from build123d import *

# Parameters (mm, degrees)
SKETCH1_R               = 10
BOSS_EXTRUDE1_DEPTH     = 35
SKETCH2_R               = 15
BOSS_EXTRUDE2_DEPTH     = 10
SKETCH3_R               = 2.5
BOSS_EXTRUDE3_DEPTH     = 5
CUT_EXTRUDE1_DEPTH      = 50
CUT_EXTRUDE1_DEPTH_BACK = 26
SKETCH7_R               = 2.5


with BuildPart() as part:
    # Sketch1 → Boss-Extrude1 (new body)
    with BuildSketch(Plane(origin=(0, 0, 0), x_dir=(1, 0, 0), z_dir=(0, 1, 0))):
        with Locations(Location((0, 0, 0), (0, 0, 270))):
            Circle(SKETCH1_R)
    extrude(amount=BOSS_EXTRUDE1_DEPTH)

    # Sketch2 → Boss-Extrude2 (add)
    with BuildSketch(Plane(origin=(0, 35, 0), x_dir=(1, 0, 0), z_dir=(0, 1, 0))):
        with Locations(Location((0, 0, 0), (0, 0, 270))):
            Circle(SKETCH2_R)
    extrude(amount=BOSS_EXTRUDE2_DEPTH)

    # Sketch3 → Boss-Extrude3 (add)
    with BuildSketch(Plane(origin=(0, 45, 0), x_dir=(1, 0, 0), z_dir=(0, 1, 0))):
        with BuildLine():
            Line((-60, 0), (-60, 12.589573297))
            Line((-60, 12.589573297), (-17.498503567, 12.589573297))
            ThreePointArc((-17.498503567, 12.589573297), (-13.964027799, 14.053601095), (-12.5, 17.588076863))
            Line((-12.5, 17.588076863), (-12.5, 60))
            Line((-12.5, 60), (12.589573297, 60))
            Line((12.589573297, 60), (12.589573297, 17.498503567))
            ThreePointArc((12.589573297, 17.498503567), (14.053601095, 13.964027799), (17.588076863, 12.5))
            Line((17.588076863, 12.5), (60, 12.5))
            Line((60, 12.5), (60, -12.589573297))
            Line((60, -12.589573297), (17.498503567, -12.589573297))
            ThreePointArc((17.498503567, -12.589573297), (13.964027799, -14.053601095), (12.5, -17.588076863))
            Line((12.5, -17.588076863), (12.5, -60))
            Line((12.5, -60), (-12.589573297, -60))
            Line((-12.589573297, -60), (-12.589573297, -17.498503567))
            ThreePointArc((-12.589573297, -17.498503567), (-14.053601095, -13.964027799), (-17.588076863, -12.5))
            Line((-17.588076863, -12.5), (-60, -12.5))
            Line((-60, -12.5), (-60, 0))
        make_face()
        with Locations(Location((0, 40, 0), (0, 0, 270))):
            Circle(SKETCH3_R, mode=Mode.SUBTRACT)
        with Locations(Location((40, 0, 0), (0, 0, 270))):
            Circle(SKETCH3_R, mode=Mode.SUBTRACT)
        with Locations(Location((0, -40, 0), (0, 0, 270))):
            Circle(SKETCH3_R, mode=Mode.SUBTRACT)
        with Locations(Location((-40, 0, 0), (0, 0, 270))):
            Circle(SKETCH3_R, mode=Mode.SUBTRACT)
    extrude(amount=BOSS_EXTRUDE3_DEPTH)

    # Sketch7 → Cut-Extrude1 (cut, two sides: drawn at the far end of the back side and taken through both)
    with BuildSketch(Plane.XY.offset(-CUT_EXTRUDE1_DEPTH_BACK)):
        with Locations(Location((0, 16.5, 0), (0, 0, 90.000000004))):
            Circle(SKETCH7_R)
    extrude(amount=CUT_EXTRUDE1_DEPTH + CUT_EXTRUDE1_DEPTH_BACK, mode=Mode.SUBTRACT)


solid = part.part
Could you check a few things on this model? Use its own coordinates, in mm. A direction names the side the tool comes from. Round coordinates to 2 decimals unless told otherwise and drop trailing zeros. Loops run counter-clockwise (first coordinate to the right, second up) from the corner with the lowest first, then second, coordinate; pieces in that order, holes last. Notation, with made-up numbers: (63.5, -23.75) - (106.5, -23.75) arc R26 cw to (106.5, 11.25) - close; hole circle Ø4 at (2.25, 64). An arc over 180 degrees is marked (long way). Write item = value, one per line.
1) Imagine slicing it at B-B (z = 0). Please give me the cut outline in (x, y), and give its area (3 significant figures).
Computed:
outline = (-60, 45) - (-42.5, 45) - (-42.5, 50) - (-60, 50) - close; (-37.5, 45) - (-15, 45) - (-15, 35) - (-10, 35) - (-10, 0) - (10, 0) - (10, 35) - (15, 35) - (15, 45) - (37.5, 45) - (37.5, 50) - (-37.5, 50) - close; (42.5, 45) - (60, 45) - (60, 50) - (42.5, 50) - close; hole circle Ø5 at (0, 16.5)
area = 1,530 mm2
2) On a 3-axis mill with a long thin cutter (end or side, diameter ignored), from which of +Z, -Z, +X, -X, +Y, -Y can I reach the whole of each face in a straight line? I mean faces 1 (the flat face through (39, 47, 12.59)), 2 (the flat face through (-38, 47, 12.5)), 3 (the flat face through (12.59, 47, -39)), 4 (the flat face through (-12.5, 47, -38)). Say none if no direction works.
Computed:
face_1 = +Z, +X, +Y, -Y
face_2 = +Z, -X, +Y, -Y
face_3 = -Z, +X, +Y, -Y
face_4 = -Z, -X, +Y, -Y
3) Imagine slicing it at A-A (x = -40). Please give me the cut outline in (y, z).
Computed:
outline = (45, -12.59) - (50, -12.59) - (50, -2.5) - (45, -2.5) - close; (45, 2.5) - (50, 2.5) - (50, 12.5) - (45, 12.5) - close
4) I need wall thicknesses on line 1 along X through (y, z) = (46.65, 0); line 2 along X through (y, z) = (47, 50.5); line 3 along Y through (x, z) = (0, 1). Which ranges of each line are inside material? Lowest first, please. Write a range as from..to.
Computed:
line_1 = -60..-42.5, -37.5..37.5, 42.5..60
line_2 = -12.59..12.5
line_3 = 0..14, 19..50
5) Imagine slicing it at D-D (y = 37). Please give me the cut outline in (x, z).
Computed:
outline = circle Ø30 at (0, 0)
6) I'm going to push flat-ended pins straight in: P1, Ø2.5, axis at x = -36.5, y = 47, coming from the +Z side; P2, Ø4, axis at y = 47, z = 49, coming from the -X side; P3, Ø6.5, axis at x = 0, z = -40, coming from the -Y side. Where does each tip first touch, or does it pass through?
Computed:
P1 = 12.5
P2 = -12.59
P3 = 45
7) If we mould it in two halves opening along Z, with no side actions, what happens to faces 5 (the cylindrical face through (-0.96, 47.46, 42.31)), 6 (the flat face through (38, 47, -12.5)), 7 (the flat face through (-10, 35, 3))? For each: pulls with the +Z half, pulls with the -Z half, needs draft (parallel to the pull), parting line crosses it, or undercut.
Computed:
face_5 = undercut
face_6 = pulls with the -Z half
face_7 = needs draft
8) Imagine slicing it at C-C (x = 0). Please give me the cut outline in (y, z), and give its area (3 significant figures).
Computed:
outline = (0, -10) - (14, -10) - (14, 10) - (0, 10) - close; (19, -10) - (35, -10) - (35, -15) - (45, -15) - (45, -37.5) - (50, -37.5) - (50, 37.5) - (45, 37.5) - (45, 15) - (35, 15) - (35, 10) - (19, 10) - close; (45, -60) - (50, -60) - (50, -42.5) - (45, -42.5) - close; (45, 42.5) - (50, 42.5) - (50, 60) - (45, 60) - close
area = 1,450 mm2
